from build123d import *

# Parameters (mm, degrees)
SKETCH2_R           = 5
BOSS_EXTRUDE1_DEPTH = 20
CUT_EXTRUDE3_DEPTH  = 15
BOSS_EXTRUDE2_DEPTH = 9.5
SKETCH6_R           = 2.85
BOSS_EXTRUDE3_DEPTH = 2.5
FILLET3_R           = 0.1


with BuildPart() as part:
    # Sketch2 → Boss-Extrude1 (new body)
    with BuildSketch(Plane(origin=(0, 0, 0), x_dir=(1, 0, 0), z_dir=(0, 1, 0))):
        with Locations(Location((0, 0, 0), (0, 0, 270))):
            Circle(SKETCH2_R)
    extrude(amount=BOSS_EXTRUDE1_DEPTH)

    # Sketch3 → Cut-Extrude3 (cut)
    with BuildSketch(Plane(origin=(0, 20, 0), x_dir=(1, 0, 0), z_dir=(0, 1, 0))):
        with BuildLine():
            Line((2.1, 1.616322988), (2.1, -1.616322988))
            ThreePointArc((2.1, -1.616322988), (-2.65, 0), (2.1, 1.616322988))
        make_face()
    extrude(amount=-CUT_EXTRUDE3_DEPTH, mode=Mode.SUBTRACT)

    # Sketch4 → Boss-Extrude2 (add)
    with BuildSketch(Plane(origin=(0, 0, 0), x_dir=(-1, 0, 0), z_dir=(0, -1, 0))):
        with BuildLine():
            Line((1.564448785, 1.95), (-1.564448785, 1.95))
            ThreePointArc((-1.564448785, 1.95), (-2.5, 0), (-1.564448785, -1.95))
            Line((-1.564448785, -1.95), (1.564448785, -1.95))
            ThreePointArc((1.564448785, -1.95), (2.5, 0), (1.564448785, 1.95))
        make_face()
    extrude(amount=BOSS_EXTRUDE2_DEPTH)

    # Sketch6 → Boss-Extrude3 (add)
    with BuildSketch(Plane.XZ):
        with Locations(Location((0, 0, 0), (0, 0, 90))):
            Circle(SKETCH6_R)
    extrude(amount=BOSS_EXTRUDE3_DEPTH)

    # Fillet3
    fillet3_edges = [part.edges().sort_by_distance(p)[0] for p in [
        (0, 20, -5),
        (-2.65, 20, 0),
    ]]
    fillet(fillet3_edges, radius=FILLET3_R)


solid = part.part
Design review of the part built by this model. Coordinates are the model's own, in mm. A direction names the side the tool comes from. Give positions to 0.01 mm unless a question says otherwise; leave off trailing zeros. Order: outer loops, then holes, each group sorted by start corner. A loop starts at its lowest first (then second) coordinate and runs counter-clockwise, first axis right, second up.
1. Mouldability with a two-part tool opening along Z and no side actions: class faces 1 (the cylindrical face through (-2.5, -6, 0)), 2 (the cylindrical face through (-2.65, 12.55, 0.09)), 3 (the flat face through (0, -9.5, 0)) as +Z half, -Z half, draft (parallel to the pull), parting line (faces both ways), or undercut.
Solution:
face 1: parting line
face 2: undercut
face 3: draft
2. Tool access review of faces 4 (the flat face through (0.2, -2.5, 2.1)), 5 (the cylindrical face through (2.5, -6, 0)), 6 (the flat face through (0, -6, 1.95)), 7 (the flat face through (2.1, 13, 0)), 8 (the flat face through (0, -6, -1.95)): name each direction out of +Z, -Z, +X, -X, +Y, -Y from which nothing blocks a thin tool from reaching the whole face with its end or side.
Solution:
face 4: -Y
face 5: +X, -Y
face 6: +Z, +X, -X, -Y
face 7: +Y
face 8: -Z, +X, -X, -Y
3. Add section A-A, the plane z = 0. State the section outline as (x, y) points, then the cut area to 3 significant figures.
Solution:
outline: (-5, 0) - (-2.85, 0) - (-2.85, -2.5) - (-2.5, -2.5) - (-2.5, -9.5) - (2.5, -9.5) - (2.5, -2.5) - (2.85, -2.5) - (2.85, 0) - (5, 0) - (5, 19.9) arc R0.1 ccw to (4.9, 20) - (2.1, 20) - (2.1, 5) - (-2.65, 5) - (-2.65, 19.9) arc R0.1 ccw to (-2.75, 20) - (-4.9, 20) arc R0.1 ccw to (-5, 19.9) - close
area: 178 mm2
4. For pin 1 Ø3.5 at (x, y) = (0.5, -7.5) entering from +Z; pin 2 Ø1.5 at (y, z) = (4.5, 2.5) entering from -X; pin 3 Ø1.4 at (x, z) = (0.5, 0) entering from +Y, all flat-tipped, find the tip position at first contact; note any pin that passes through.
Solution:
pin 1: stops at z = 1.95
pin 2: stops at x = -4.68
pin 3: stops at y = 5
5. Add section B-B, the plane y = 17.5. State the section outline as (x, z) points.
Solution:
outline: circle Ø10 at (0, 0); hole (2.1, -1.62) - (2.1, 1.62) arc R2.65 ccw (long way) to start
6. To check wall thickness, follow L1, parallel to Y at x = 3, z = -2.5; L2, parallel to Z at x = 0.25, y = -5.5; L3, parallel to Z at x = 0.5, y = 11.75. State the ranges of each line that lie inside material, in increasing order.
Solution:
L1: y = 0 to 20
L2: z = -1.95 to 1.95
L3: z = -4.97 to -2.6, 2.6 to 4.97
